The drawing under review shows one solid part. Ordinate dimensions are in mm from its lowest x, y, z. A direction names the side the tool comes from. Coordinates: 2 decimals unless noted, no trailing zeros. Write each loop counter-clockwise with the first axis right and the second up, starting at its lowest first coordinate (ties: lowest second). Pieces come first, ordered by that corner, then holes. Notation, with made-up numbers: (78, 36) -> (120, 36) arc R20 cw to (120, 69) -> close; hole circle Ø1 at (76, 57.5). An arc over 180 degrees is marked (long way). One line per item, written item: value. Start each with the question number.
1) Add section C-C (z = 97). State the section outline as (x, y) points, and give its area (3 significant figures).
2) Add section A-A (z = 38.1). State the section outline as (x, y) points.
3) Mouldability with a two-part tool opening along Y and no side actions: class the marked faces 1, 2, 3 and 4 as released by +Y, released by -Y, zero draft, split by the parting line, or undercut.
4) Add section B-B (x = 15.75). State the section outline as (y, z) points.
5) Machinability: for the marked faces 5 and 6, which of the approach directions +Z, -Z, +X, -X, +Y, -Y give a long, thin tool a straight path to every point of the face, cutting with its end or side? Answer none if there is none.
6) For probe 1 along X at (y, z) = (11, 54); probe 2 along Y at (x, z) = (0.45, 88.9), list the stretches that pass through material, from the lowest coordinate up. Write a range as from..to.
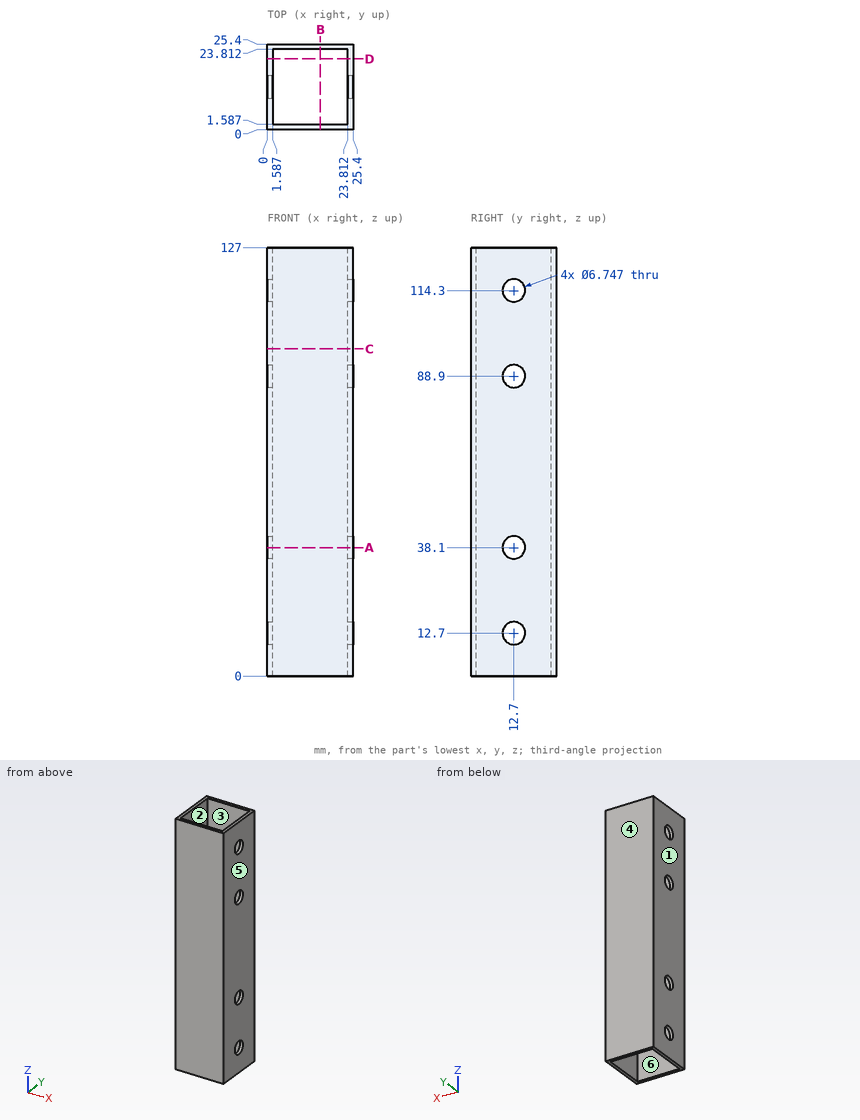
Numbers:
1. outline: (0, 0) -> (25.4, 0) -> (25.4, 25.4) -> (0, 25.4) -> close; hole (1.59, 1.59) -> (23.81, 1.59) -> (23.81, 23.81) -> (1.59, 23.81) -> close
1. area: 151 mm²
2. outline: (0, 0) -> (25.4, 0) -> (25.4, 9.33) -> (23.81, 9.33) -> (23.81, 1.59) -> (1.59, 1.59) -> (1.59, 9.33) -> (0, 9.33) -> close; (0, 16.07) -> (1.59, 16.07) -> (1.59, 23.81) -> (23.81, 23.81) -> (23.81, 16.07) -> (25.4, 16.07) -> (25.4, 25.4) -> (0, 25.4) -> close
3. face 1: zero draft
3. face 2: undercut
3. face 3: undercut
3. face 4: released by +Y
4. outline: (0, 0) -> (1.59, 0) -> (1.59, 127) -> (0, 127) -> close; (23.81, 0) -> (25.4, 0) -> (25.4, 127) -> (23.81, 127) -> close
5. face 5: +Z, -Z, +X, +Y, -Y
5. face 6: +Z, -Z
6. probe 1: 0..1.59, 23.81..25.4
6. probe 2: 0..9.33, 16.07..25.4
